from build123d import *

# Parameters (mm, degrees)
F0_W     = 80
F0_H     = 50
F1_DEPTH = 50
F2_R     = 10
F3_DEPTH = 25
F4_W     = 10
F4_H     = 10
F5_DEPTH = 5
F6_R     = 7.5
F7_DEPTH = 5


with BuildPart() as f1:
    # F0 (on Top) → F1 (new body)
    with BuildSketch(Plane.XY):
        Rectangle(F0_W, F0_H)
    extrude(amount=F1_DEPTH)

    # F2 (on face) → F3 (join)
    with BuildSketch(Plane.XZ.offset(25)):
        with Locations((0, 25)):
            Circle(F2_R)
    extrude(amount=F3_DEPTH)

    # F4 (on face) → F5 (cut)
    with BuildSketch(Plane.XZ.offset(50)):
        with Locations((0, 25)):
            Rectangle(F4_W, F4_H)
    extrude(amount=-F5_DEPTH, mode=Mode.SUBTRACT)

    # F6 (on face) → F7 (join)
    with BuildSketch(Plane.XY.offset(50)):
        with Locations((-27.5, -12.5)):
            Circle(F6_R)
    extrude(amount=F7_DEPTH)


solid = f1.part
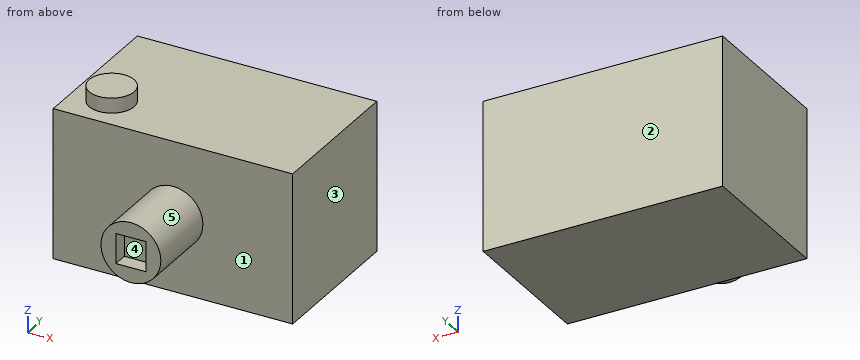
Part model, mm, in its own coordinate system. Face numbers are marked on the shaded views. A direction names the side the tool comes from. Give positions to 0.01 mm unless a question says otherwise; leave off trailing zeros. Order: outer loops, then holes, each group sorted by start corner. A loop starts at its lowest first (then second) coordinate and runs counter-clockwise, first axis right, second up. Notation, with made-up numbers: (34, -21) - (89, -21) arc R23 cw to (89, 10) - close; hole circle Ø6 at (66.25, 77.25). An arc over 180 degrees is marked (long way). One line per question, with ' | ' between items.
1. Which spindle directions (+Z, -Z, +X, -X, +Y, -Y) get a long thin tool onto all of the face, cutting with end or side? Do the marked faces 1 and 2. Say none if no direction does.
Filled in:
face 1: -Y | face 2: +Z, -Z, +X, -X, +Y
2. Drop flat-ended pins along their axis: P1, Ø2.5, axis at x = -1, y = -46.5, coming from the -Z side; P2, Ø4, axis at y = -46.5, z = 25, coming from the +X side; P3, Ø4, axis at x = -5.5, y = -12.5, coming from the +Z side; P4, Ø4, axis at x = -5, y = -3.5, coming from the -Z side. Give the stop position or say it passes through.
Filled in:
P1: z = 15 | P2: x = 10 | P3: z = 50 | P4: z = 0
3. Band-saw the part on C-C on y = -12.5. List the corners of the cut face in (x, z), then the cut area to 4 significant figures.
Filled in:
outline: (-40, 0) - (40, 0) - (40, 50) - (-20, 50) - (-20, 55) - (-35, 55) - (-35, 50) - (-40, 50) - close | area: 4,075 mm²
4. Band-saw the part on A-A on x = -27.5. List the corners of the cut face in (y, z).
Filled in:
outline: (-25, 0) - (25, 0) - (25, 50) - (-5, 50) - (-5, 55) - (-20, 55) - (-20, 50) - (-25, 50) - close
5. Pull direction Z, two halves, no side cores. Call the marked faces 3, 4 and 5: +Z half, -Z half, draft (parallel to the pull), parting line (faces both ways), or undercut.
Filled in:
face 3: draft | face 4: undercut | face 5: parting line
6. Drill centre lines: probe 1 along Y at (x, z) = (23.5, 31.5); probe 2 along Z at (x, y) = (-21.5, 0.5); probe 3 along X at (y, z) = (-37.5, 29). Where is each one in solid material? Low to high.
Filled in:
probe 1: -25 to 25 | probe 2: 0 to 50 | probe 3: -9.17 to 9.17
7. Band-saw the part on B-B on z = 25. List the corners of the cut face in (x, y).
Filled in:
outline: (-40, -25) - (-10, -25) - (-10, -50) - (-5, -50) - (-5, -45) - (5, -45) - (5, -50) - (10, -50) - (10, -25) - (40, -25) - (40, 25) - (-40, 25) - close
8. Band-saw the part on D-D on x = 0. List the corners of the cut face in (y, z).
Filled in:
outline: (-50, 15) - (-25, 15) - (-25, 0) - (25, 0) - (25, 50) - (-25, 50) - (-25, 35) - (-50, 35) - (-50, 30) - (-45, 30) - (-45, 20) - (-50, 20) - close
